from build123d import *

# Parameters (mm, degrees)
SKETCH1_R               = 6
BOSS_EXTRUDE1_DEPTH     = 23
SKETCH2_R               = 3
BOSS_EXTRUDE2_DEPTH     = 10
CHAMFER1_SIZE           = 0.5
CHAMFER2_SIZE           = 0.25
CUT_EXTRUDE1_DEPTH      = 35.073450075
CUT_EXTRUDE1_DEPTH_BACK = 35.073450075
SKETCH4_R               = 1.25


with BuildPart() as part:
    # Sketch1 → Boss-Extrude1 (new body)
    with BuildSketch(Plane.XY):
        Circle(SKETCH1_R)
    extrude(amount=BOSS_EXTRUDE1_DEPTH)

    # Sketch2 → Boss-Extrude2 (add)
    with BuildSketch(Plane.XY.offset(23)):
        Circle(SKETCH2_R)
    extrude(amount=BOSS_EXTRUDE2_DEPTH)

    # Chamfer1
    chamfer1_edges = [part.edges().sort_by_distance(p)[0] for p in [
        (-6, 0, 0),
        (-6, 0, 23),
    ]]
    chamfer(chamfer1_edges, length=CHAMFER1_SIZE)

    # Chamfer2
    chamfer2_edges = [part.edges().sort_by_distance(p)[0] for p in [
        (-3, 0, 33),
    ]]
    chamfer(chamfer2_edges, length=CHAMFER2_SIZE)

    # Sketch4 → Cut-Extrude1 (cut, two sides: drawn at the far end of the back side and taken through both)
    with BuildSketch(Plane(origin=(0, 0, 0), x_dir=(0, 0, -1), z_dir=(1, 0, 0)).offset(-CUT_EXTRUDE1_DEPTH_BACK)):
        with Locations((-5, 0)):
            Circle(SKETCH4_R)
    extrude(amount=CUT_EXTRUDE1_DEPTH + CUT_EXTRUDE1_DEPTH_BACK, mode=Mode.SUBTRACT)


solid = part.part
The model under review builds one solid part; all positions refer to its coordinate system, in mm. A direction names the side the tool comes from. Round coordinates to 2 decimals unless told otherwise and drop trailing zeros. Order: outer loops, then holes, each group sorted by start corner. A loop starts at its lowest first (then second) coordinate and runs counter-clockwise, first axis right, second up. Notation, with made-up numbers: (-15, 35.5) -> (2, 35.5) arc R17 ccw to (2, 52.5) -> close; hole circle Ø11 at (60, 21). An arc over 180 degrees is marked (long way). Return JSON: item names as keys, results as strings.
1. Take a section at B-B (y = 0). Write out the cut boundary in (x, z), then the cut area to 3 significant figures.
Answer block:
{"outline": "(-6, 0.5) -> (-5.5, 0) -> (5.5, 0) -> (6, 0.5) -> (6, 3.75) -> (-6, 3.75) -> close; (-6, 6.25) -> (6, 6.25) -> (6, 22.5) -> (5.5, 23) -> (3, 23) -> (3, 32.75) -> (2.75, 33) -> (-2.75, 33) -> (-3, 32.75) -> (-3, 23) -> (-5.5, 23) -> (-6, 22.5) -> close", "area": "305 mm²"}
2. For faces 1 (the face through (0, 0, 33)), 2 (the face through (-3, 0, 28)), list the 3-axis set-ups (+Z, -Z, +X, -X, +Y, -Y) from which the entire face can be reached by the end or side of a thin tool; tool diameter is ignored.
Answer block:
{"face 1": "+Z, +X, -X, +Y, -Y", "face 2": "+Z"}
3. The part is to be moulded in two halves that separate along Y. For faces 3 (the face through (2.4, -2.4, 23)), 4 (the face through (-0.08, 0.05, 6.25)), 5 (the face through (5.723, 1.802, 11.346)), say which applies: +Y half, -Y half, draft (parallel to the pull), parting line (faces both ways), or undercut.
Answer block:
{"face 3": "draft", "face 4": "undercut", "face 5": "parting line"}
4. Take a section at C-C (z = 2). Write out the cut boundary in (x, y).
Answer block:
{"outline": "circle Ø12 at (0, 0)"}
5. Insertion check: P1, Ø1, axis at x = 4.5, z = 11.5, coming from the +Y side; P2, Ø4, axis at y = 0, z = 5, coming from the -X side; P3, Ø2, axis at x = -4, z = 16, coming from the +Y side. Each pin has a flat end and moves straight along its axis. Give the tip position at first contact, or say it passes through.
Answer block:
{"P1": "stops at y = 4.47", "P2": "stops at x = -6", "P3": "stops at y = 5.2"}
6. For L1, parallel to Z at x = -0.75, y = 0; L2, parallel to Y at x = -0.25, z = 5; L3, parallel to Z at x = -3.5, y = -3, list the stretches that pass through material, from the lowest coordinate up. Write a range as [from, to].
Answer block:
{"L1": "z = [0, 3.75], [6.25, 33]", "L2": "y = [-5.99, -1.25], [1.25, 5.99]", "L3": "z = [0, 23]"}
7. Take a section at A-A (x = 0). Write out the cut boundary in (y, z).
Answer block:
{"outline": "(-6, 0.5) -> (-5.5, 0) -> (5.5, 0) -> (6, 0.5) -> (6, 22.5) -> (5.5, 23) -> (3, 23) -> (3, 32.75) -> (2.75, 33) -> (-2.75, 33) -> (-3, 32.75) -> (-3, 23) -> (-5.5, 23) -> (-6, 22.5) -> close; hole circle Ø2.5 at (0, 5)"}
